Input: part model. Units: mm. Frame: model coordinates. A direction names the side the tool comes from. Give positions to 0.01 mm unless a question says otherwise; leave off trailing zeros. Loops run counter-clockwise (first coordinate to the right, second up) from the corner with the lowest first, then second, coordinate; pieces in that order, holes last. Notation, with made-up numbers: M 76,76.5 L 120,76.5 A14 ccw 120,85.5 Z; hole C -7,0 d11. An arc over 180 degrees is marked long. Use a Markdown table: item, result. Add a question column.
from build123d import *

# Parameters (mm, degrees)
EXTRUDE1_DEPTH     = 19.05
EXTRUDE4_DEPTH     = 2.921
SKETCH5_W          = 47.9552
SKETCH5_H          = 2.921
EXTRUDE5_DEPTH     = 19.05
FILLET1_R          = 4.064
FILLET2_START      = 790
FILLET2_2_DEPTH    = 44.1360001
SKETCH6_R          = 2.413
CUT_EXTRUDE1_DEPTH = 5.842


with BuildPart() as part:
    # Sketch2 → Extrude1 (new body)
    with BuildSketch(Plane.XY):
        with BuildLine():
            Line((356.4255, 790.321), (306.8955, 790.321))
            Line((306.8955, 790.321), (306.8955, 787.4))
            Line((306.8955, 787.4), (356.4255, 787.4))
            ThreePointArc((356.4255, 787.4), (359.837997326, 788.813502674), (361.2515, 792.226))
            Line((361.2515, 792.226), (361.2515, 834.136))
            ThreePointArc((361.2515, 834.136), (361.586276949, 834.944223051), (362.3945, 835.279))
            Line((362.3945, 835.279), (376.936, 835.279))
            ThreePointArc((376.936, 835.279), (377.744223051, 834.944223051), (378.079, 834.136))
            Line((378.079, 834.136), (378.079, 825.4492))
            Line((378.079, 825.4492), (381, 825.4492))
            Line((381, 825.4492), (381, 834.136))
            ThreePointArc((381, 834.136), (379.809681959, 837.009681959), (376.936, 838.2))
            Line((376.936, 838.2), (362.3945, 838.2))
            ThreePointArc((362.3945, 838.2), (359.520818041, 837.009681959), (358.3305, 834.136))
            Line((358.3305, 834.136), (358.3305, 792.226))
            ThreePointArc((358.3305, 792.226), (357.772538418, 790.878961582), (356.4255, 790.321))
        make_face()
    extrude(amount=EXTRUDE1_DEPTH)



with BuildPart() as body_2:
    # Sketch3 → Extrude4 (new body)
    with BuildSketch(Plane.XY):
        Polygon((306.8955, 793.242), (351.5995, 829.945), (361.2515, 829.945), (361.2515, 796.82051965), (354.8507, 796.82051965), (354.8507, 790.321), (306.8955, 790.321), align=None)
    extrude(amount=-EXTRUDE4_DEPTH)


with BuildPart() as part_1:
    add(part.part)

    add(body_2.part)  # Extrude5 merges body 2
    # Sketch5 → Extrude5 (add)
    with BuildSketch(Plane.XY):
        with Locations((330.8731, 791.7815)):
            Rectangle(SKETCH5_W, SKETCH5_H)
    extrude(amount=EXTRUDE5_DEPTH)

    # Fillet1
    # the kernel refuses this fillet: 4.064 mm, written as the material it takes off along each edge
    with BuildSketch(Plane(origin=(364.600586858, 790.321, -2.921), x_dir=(0, 0, 1), z_dir=(-1, 0, 0))) as fillet1_piece_1:
        with BuildLine():
            CenterArc((4.064, 3.899954743), FILLET1_R, 180, 73.665177219)
            Line((0, 3.899954743), (-0.08128, 3.899954743))
            Line((-0.08128, 3.899954743), (-0.08128, 0))
            Line((-0.08128, 0), (0, -0.08128))
            ThreePointArc((0, -0.08128), (1.4605, -0.08128), (2.89814, -0.077999095))
            Line((2.89814, -0.077999095), (2.921, 0))
        make_face()
    extrude(amount=67.454973717, mode=Mode.SUBTRACT)

    # Fillet2: read off the stored shape, not the designer's step
    # Fillet2 outline → Fillet2 (revolve, cut)
    with BuildSketch(Plane(origin=(362.3945, 834.136, 0), x_dir=(1, 0, 0), z_dir=(0, -1, 0))):
        with BuildLine():
            Line((1.143, 0), (1.307045257, 0))
            ThreePointArc((1.307045257, 0), (1.184220359, 0.565643991), (1.143, 1.143))
            Line((1.143, 1.143), (1.143, 0))
        make_face()
    revolve(axis=Axis((362.3945, 834.136, 0), (0, 0, 1)), mode=Mode.SUBTRACT)

    # Fillet2 2 outline → Fillet2 2 (cut)
    with BuildSketch(Plane(origin=(0, 0, 0), x_dir=(1, 0, 0), z_dir=(0, 1, 0)).offset(FILLET2_START)):
        with BuildLine():
            Line((361.2515, 2.921), (357.1875, 2.921))
            ThreePointArc((357.1875, 2.921), (360.061181959, 1.730681959), (361.2515, -1.143))
            Line((361.2515, -1.143), (361.2515, 2.921))
        make_face()
    extrude(amount=FILLET2_2_DEPTH, mode=Mode.SUBTRACT)

    # Sketch6 → Cut-Extrude1 (cut)
    with BuildSketch(Plane.XZ.offset(-787.4)):
        with Locations(Location((313.2455, 9.525, 0), (0, 0, 270))):
            Circle(SKETCH6_R)
        with Locations(Location((338.6455, 9.525, 0), (0, 0, 270))):
            Circle(SKETCH6_R)
    extrude(amount=-CUT_EXTRUDE1_DEPTH, mode=Mode.SUBTRACT)


solid = part_1.part
1) Contact query for flat-ended pins moving along their axis: P1, Ø1.5, axis at x = 380, z = 8.5, coming from the -Y side; P2, Ø3, axis at x = 336, y = 792.5, coming from the -Z side (3 decimals); P3, Ø1, axis at x = 359.5, z = 5, coming from the +Y side; P4, Ø4, axis at x = 313.25, z = 9.52, coming from the +Y side. Output: stop coordinate, or through.
2) Section query A-A, the plane z = 8. Return the cut outline in (x, y) (1 decimal), and give its area (3 significant figures).
3) Section query C-C, the plane x = 319. Return the cut outline in (y, z), and give its area (3 significant figures).
4) Section query D-D, the plane y = 804. Return the cut outline in (x, z).
5) Section query B-B, the plane y = 796. Return the cut outline in (x, z), and give its area (3 significant figures).
6) Pull-direction query (Z, two-part tool) for faces 1 (the flat face through (331, 793.242, 9)), 2 (the flat face through (336, 789, 0)), 3 (the flat face through (347, 792, 19.05)), 4 (the cylindrical face through (315.638, 790.28, 9.839)); classes: pulls with the +Z half, pulls with the -Z half, needs draft (parallel to the pull), parting line crosses it, or undercut.
7) Ray query, line 1 (X direction, y = 832.5, z = 1.75); line 2 (X direction, y = 793, z = 12.5); line 3 (Y direction, x = 338.5, z = 3.5). Return the intervals inside material, ascending. Write a range as [from, to].
8) Reachability of faces 5 (the flat face through (356, 829.945, -1)), 6 (the cylindrical face through (357.787, 790.894, 9.392)), 7 (the flat face through (378.079, 830, 9)), 8 (the flat face through (357, 796.821, -1)) from +Z, -Z, +X, -X, +Y, -Y: full face, straight path, thin tool, end or side. Return the list, or none.
Entries:
| question | item | result |
|---|---|---|
| 1 | P1 | stops at y = 825.45 |
| 1 | P2 | stops at z = -2.915 |
| 1 | P3 | stops at y = 837.42 |
| 1 | P4 | passes through |
| 2 | outline | M 306.9,787.4 L 311.4,787.4 L 311.4,793.2 L 306.9,793.2 Z; M 315.1,787.4 L 336.8,787.4 L 336.8,793.2 L 315.1,793.2 Z; M 340.5,787.4 L 356.4,787.4 A4.8 ccw 361.3,792.2 L 361.3,834.1 A1.1 cw 362.4,835.3 L 376.9,835.3 A1.1 cw 378.1,834.1 L 378.1,825.4 L 381,825.4 L 381,834.1 A4.1 ccw 376.9,838.2 L 362.4,838.2 A4.1 ccw 358.3,834.1 L 358.3,792.2 A1.9 cw 356.4,790.3 L 354.9,790.3 L 354.9,793.2 L 340.5,793.2 Z |
| 2 | area | 471 mm² |
| 3 | outline | M 787.4,0 L 790.32,0 A4.06 ccw 794.22,-2.92 L 803.18,-2.92 L 803.18,0 L 793.24,0 L 793.24,19.05 L 787.4,19.05 Z |
| 3 | area | 146 mm² |
| 4 | outline | M 320,-2.92 L 357.19,-2.92 A4.06 ccw 361.25,1.14 L 361.25,19.05 L 358.33,19.05 L 358.33,0 L 320,0 Z |
| 5 | outline | M 310.25,-2.92 L 354.85,-2.92 L 354.85,0 L 310.25,0 Z; M 358.33,0 L 361.09,0 A4.06 ccw 361.25,1.14 L 361.25,19.05 L 358.33,19.05 Z |
| 5 | area | 186 mm² |
| 6 | face 1 | needs draft |
| 6 | face 2 | pulls with the -Z half |
| 6 | face 3 | pulls with the +Z half |
| 6 | face 4 | undercut |
| 7 | line 1 | x = [358.33, 361.25], [378.08, 381] |
| 7 | line 2 | x = [306.9, 354.85], [358.33, 361.25] |
| 7 | line 3 | y = [787.4, 793.24] |
| 8 | face 5 | -Z, +X, -X, +Y |
| 8 | face 6 | +Z, -Z, +Y |
| 8 | face 7 | +Z, -Z, -Y |
| 8 | face 8 | -Z, +X, -Y |
